Design review of the part built by this model. Coordinates are the model's own, in mm. Face numbers are marked on the shaded views. A direction names the side the tool comes from. Coordinates: 2 decimals unless noted, no trailing zeros. Loops run counter-clockwise (first coordinate to the right, second up) from the corner with the lowest first, then second, coordinate; pieces in that order, holes last. Notation, with made-up numbers: (25, 81) - (42, 81) arc R21 ccw to (42, 110) - close; hole circle Ø5 at (87, -22.5). An arc over 180 degrees is marked (long way). Use one line per item in the form item = value. Start each with the question number.
(1) Tool access review of the marked faces 5, 6, 7 and 8: name each direction out of +Z, -Z, +X, -X, +Y, -Y from which nothing blocks a thin tool from reaching the whole face with its end or side.
(2) For L1, parallel to X at y = -45.5, z = -65; L2, parallel to X at y = -57.5, z = 21; L3, parallel to Z at x = 291.5, y = -2, list the stretches that pass through material, from the lowest coordinate up.
(3) Clearance check with flat-ended pins moving along their axes: pin 1 Ø14 at (x, z) = (161, 48) entering from -Y; pin 2 Ø6 at (x, y) = (159.5, -37) entering from +Z; pin 3 Ø14 at (x, y) = (423, 39.5) entering from -Z. State where each tip first meets the part, or that it passes through.
(4) Add section C-C (z = 0). State the section outline as (x, y) points.
(5) Add section B-B (y = 0). State the section outline as (x, z) points.
(6) Add section D-D (x = 76.5). State the section outline as (y, z) points.
(7) The part is to be moulded in two halves that separate along X. For the marked faces 1, 2, 3 and 4, say which applies: pulls with the +X half, pulls with the -X half, needs draft (parallel to the pull), parting line crosses it, or undercut.
(8) Add section A-A (x = 245). State the section outline as (y, z) points (3 decimals).
```python
from build123d import *

# Parameters (mm, degrees)
F0_R          = 63.5
F1_DEPTH      = 152.4
F2_R          = 63.5
F3_DEPTH      = 12.7
F4_R          = 50.8
F4_R_2        = 6.35
F5_DEPTH      = 254
F6_R          = 50.8
F7_DEPTH      = 12.7
F8_W          = 148.7337000847
F8_H          = 72.5575238466
F9_DEPTH      = 76.2
F9_DEPTH_BACK = 6.35
F10_R         = 63.5
F11_DEPTH     = 25.4


with BuildPart() as f1:
    # F0 (on Right) → F1 (new body)
    with BuildSketch(Plane.YZ):
        Circle(F0_R)
    extrude(amount=F1_DEPTH)

    # F2 (on face) → F3 (join)
    with BuildSketch(Plane.YZ.offset(152.4)):
        with BuildLine():
            ThreePointArc((-69.85, 32.3787739113), (-70.0280530831, 30.5456868066), (-70.5555555556, 28.7811323656))
            ThreePointArc((-70.5555555556, 28.7811323656), (-76.2, 0), (-70.5555555556, -28.7811323656))
            ThreePointArc((-70.5555555556, -28.7811323656), (-70.0280530831, -30.5456868066), (-69.85, -32.3787739113))
            Line((-69.85, -32.3787739113), (-69.85, -60.325))
            ThreePointArc((-69.85, -60.325), (-67.0601920908, -67.0601920908), (-60.325, -69.85))
            Line((-60.325, -69.85), (-32.3787739113, -69.85))
            ThreePointArc((-32.3787739113, -69.85), (-30.5456868066, -70.0280530831), (-28.7811323656, -70.5555555556))
            ThreePointArc((-28.7811323656, -70.5555555556), (0, -76.2), (28.7811323656, -70.5555555556))
            ThreePointArc((28.7811323656, -70.5555555556), (30.5456868066, -70.0280530831), (32.3787739113, -69.85))
            Line((32.3787739113, -69.85), (60.325, -69.85))
            ThreePointArc((60.325, -69.85), (67.0601920908, -67.0601920908), (69.85, -60.325))
            Line((69.85, -60.325), (69.85, -32.3787739113))
            ThreePointArc((69.85, -32.3787739113), (70.0280530831, -30.5456868066), (70.5555555556, -28.7811323656))
            ThreePointArc((70.5555555556, -28.7811323656), (76.2, 0), (70.5555555556, 28.7811323656))
            ThreePointArc((70.5555555556, 28.7811323656), (70.0280530831, 30.5456868066), (69.85, 32.3787739113))
            Line((69.85, 32.3787739113), (69.85, 60.325))
            ThreePointArc((69.85, 60.325), (67.0601920908, 67.0601920908), (60.325, 69.85))
            Line((60.325, 69.85), (32.3787739113, 69.85))
            ThreePointArc((32.3787739113, 69.85), (30.5456868066, 70.0280530831), (28.7811323656, 70.5555555556))
            ThreePointArc((28.7811323656, 70.5555555556), (0, 76.2), (-28.7811323656, 70.5555555556))
            ThreePointArc((-28.7811323656, 70.5555555556), (-30.5456868066, 70.0280530831), (-32.3787739113, 69.85))
            Line((-32.3787739113, 69.85), (-60.325, 69.85))
            ThreePointArc((-60.325, 69.85), (-67.0601920908, 67.0601920908), (-69.85, 60.325))
            Line((-69.85, 60.325), (-69.85, 32.3787739113))
        make_face()
        Circle(F2_R, mode=Mode.SUBTRACT)
        Circle(F2_R)
    extrude(amount=F3_DEPTH)

    # F4 (on face) → F5 (join)
    with BuildSketch(Plane.YZ.offset(165.1)):
        Circle(F4_R)
        with Locations((60.325, 60.325)):
            Circle(F4_R_2)
        with Locations((60.325, -60.325)):
            Circle(F4_R_2)
        with Locations((-60.325, -60.325)):
            Circle(F4_R_2)
        with Locations((-60.325, 60.325)):
            Circle(F4_R_2)
    extrude(amount=F5_DEPTH)

    # F6 (on face) → F7 (join)
    with BuildSketch(Plane.YZ.offset(419.1)):
        with BuildLine():
            ThreePointArc((-69.85, 32.3787739113), (-70.0280530831, 30.5456868066), (-70.5555555556, 28.7811323656))
            ThreePointArc((-70.5555555556, 28.7811323656), (-76.2, 0), (-70.5555555556, -28.7811323656))
            ThreePointArc((-70.5555555556, -28.7811323656), (-70.0280530831, -30.5456868066), (-69.85, -32.3787739113))
            Line((-69.85, -32.3787739113), (-69.85, -60.325))
            ThreePointArc((-69.85, -60.325), (-67.0601920908, -67.0601920908), (-60.325, -69.85))
            Line((-60.325, -69.85), (-32.3787739113, -69.85))
            ThreePointArc((-32.3787739113, -69.85), (-30.5456868066, -70.0280530831), (-28.7811323656, -70.5555555556))
            ThreePointArc((-28.7811323656, -70.5555555556), (0, -76.2), (28.7811323656, -70.5555555556))
            ThreePointArc((28.7811323656, -70.5555555556), (30.5456868066, -70.0280530831), (32.3787739113, -69.85))
            Line((32.3787739113, -69.85), (60.325, -69.85))
            ThreePointArc((60.325, -69.85), (67.0601920908, -67.0601920908), (69.85, -60.325))
            Line((69.85, -60.325), (69.85, -32.3787739113))
            ThreePointArc((69.85, -32.3787739113), (70.0280530831, -30.5456868066), (70.5555555556, -28.7811323656))
            ThreePointArc((70.5555555556, -28.7811323656), (76.2, 0), (70.5555555556, 28.7811323656))
            ThreePointArc((70.5555555556, 28.7811323656), (70.0280530831, 30.5456868066), (69.85, 32.3787739113))
            Line((69.85, 32.3787739113), (69.85, 60.325))
            ThreePointArc((69.85, 60.325), (67.0601920908, 67.0601920908), (60.325, 69.85))
            Line((60.325, 69.85), (32.3787739113, 69.85))
            ThreePointArc((32.3787739113, 69.85), (30.5456868066, 70.0280530831), (28.7811323656, 70.5555555556))
            ThreePointArc((28.7811323656, 70.5555555556), (0, 76.2), (-28.7811323656, 70.5555555556))
            ThreePointArc((-28.7811323656, 70.5555555556), (-30.5456868066, 70.0280530831), (-32.3787739113, 69.85))
            Line((-32.3787739113, 69.85), (-60.325, 69.85))
            ThreePointArc((-60.325, 69.85), (-67.0601920908, 67.0601920908), (-69.85, 60.325))
            Line((-69.85, 60.325), (-69.85, 32.3787739113))
        make_face()
        Circle(F6_R, mode=Mode.SUBTRACT)
        Circle(F6_R)
    extrude(amount=F7_DEPTH)

    # F8 (on face) → F9 (join, two sides)
    with BuildSketch(Plane.XY.offset(69.85)) as f9_sk:
        with Locations((292.1, 36.2787619233)):
            Rectangle(F8_W, F8_H)
        with Locations((292.1, -36.2787619233)):
            Rectangle(F8_W, F8_H)
    extrude(amount=F9_DEPTH)
    extrude(f9_sk.sketch, amount=-F9_DEPTH_BACK)

    # F10 (on face) → F11 (join)
    with BuildSketch(Plane.YZ.offset(431.8)):
        Circle(F10_R)
    extrude(amount=F11_DEPTH)


solid = f1.part
```
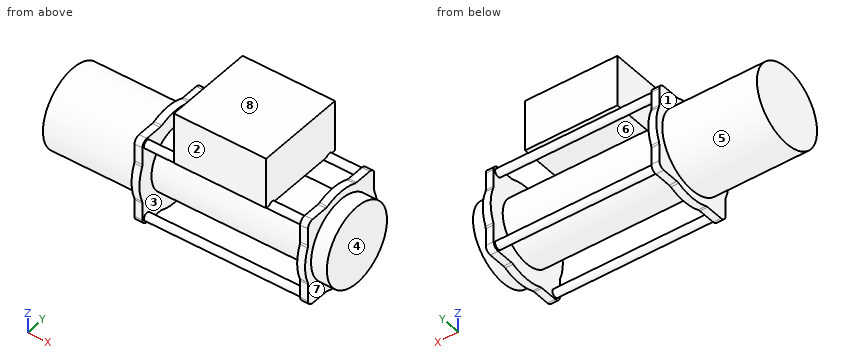
Computed values:
q1.face_5 = -X
q1.face_6 = none
q1.face_7 = +X
q1.face_8 = +Z, +X, -X, +Y, -Y
q2.L1 = 152.4 to 165.1, 419.1 to 431.8
q2.L2 = 0 to 165.1, 419.1 to 457.2
q2.L3 = -50.76 to 50.76, 63.5 to 146.05
q3.pin_1 = -69.85
q3.pin_2 = 69.85
q3.pin_3 = -69.85
q4.outline = (0, -63.5) - (152.4, -63.5) - (152.4, -76.2) - (165.1, -76.2) - (165.1, -50.8) - (419.1, -50.8) - (419.1, -76.2) - (431.8, -76.2) - (431.8, -63.5) - (457.2, -63.5) - (457.2, 63.5) - (431.8, 63.5) - (431.8, 76.2) - (419.1, 76.2) - (419.1, 50.8) - (165.1, 50.8) - (165.1, 76.2) - (152.4, 76.2) - (152.4, 63.5) - (0, 63.5) - close
q5.outline = (0, -63.5) - (152.4, -63.5) - (152.4, -76.2) - (165.1, -76.2) - (165.1, -50.8) - (419.1, -50.8) - (419.1, -76.2) - (431.8, -76.2) - (431.8, -63.5) - (457.2, -63.5) - (457.2, 63.5) - (431.8, 63.5) - (431.8, 76.2) - (419.1, 76.2) - (419.1, 50.8) - (165.1, 50.8) - (165.1, 76.2) - (152.4, 76.2) - (152.4, 63.5) - (0, 63.5) - close; (217.73, 63.5) - (366.47, 63.5) - (366.47, 146.05) - (217.73, 146.05) - close
q6.outline = circle Ø127 at (0, 0)
q7.face_1 = pulls with the -X half
q7.face_2 = needs draft
q7.face_3 = undercut
q7.face_4 = pulls with the +X half
q8.outline = (-72.558, 63.5) - (-65.824, 63.5) arc R6.35 ccw (long way) to (-54.826, 63.5) - (54.826, 63.5) arc R6.35 ccw (long way) to (65.824, 63.5) - (72.558, 63.5) - (72.558, 146.05) - (-72.558, 146.05) - close; circle Ø12.7 at (-60.325, -60.325); circle Ø101.6 at (0, 0); circle Ø12.7 at (60.325, -60.325)
